from build123d import *

# Parameters (mm, degrees)
EXTRUDE_3_DEPTH    = 3
SKETCH1_W          = 15
SKETCH1_H          = 40
SKETCH1_W_2        = 3
SKETCH1_H_2        = 20
CUT_EXTRUDE1_DEPTH = 10
FILLET1_R          = 15


with BuildPart() as part:
    # Эскиз4 → Бобышка-Вытянуть3 (new body)
    with BuildSketch(Plane(origin=(0, 0, 0), x_dir=(1, 0, 0), z_dir=(0, 1, 0))):
        Polygon((98, 0), (98, 110), (58, 110), (58, 107), (55, 107), (52, 107), (52, 110), (0, 110), (0, 58), (3, 58), (3, 55), (3, 52), (0, 52), (0, 0), (52, 0), (52, 3), (55, 3), (58, 3), (58, 0), align=None)
    extrude(amount=EXTRUDE_3_DEPTH)

    # Sketch1 → Cut-Extrude1 (cut)
    with BuildSketch(Plane(origin=(0, 3, 0), x_dir=(1, 0, 0), z_dir=(0, 1, 0))):
        with Locations((26.5, 55)):
            Rectangle(SKETCH1_W, SKETCH1_H)
        with Locations((55, 55)):
            Rectangle(SKETCH1_W_2, SKETCH1_H_2)
    extrude(amount=-CUT_EXTRUDE1_DEPTH, mode=Mode.SUBTRACT)

    # Fillet1
    fillet1_edges = [part.edges().sort_by_distance(p)[0] for p in [
        (0, 1.5, 0),
        (0, 1.5, -110),
    ]]
    fillet(fillet1_edges, radius=FILLET1_R)


solid = part.part
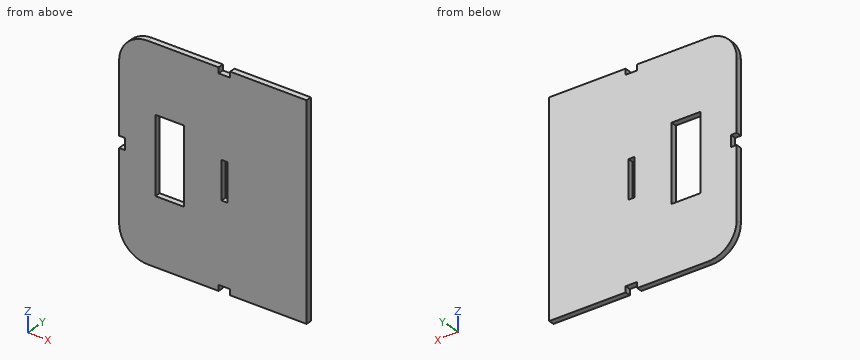
CAD build for the part. Positions are in the model's coordinates, mm. Coordinates: 2 decimals unless noted, no trailing zeros. Write each loop counter-clockwise with the first axis right and the second up, starting at its lowest first coordinate (ties: lowest second). Pieces come first, ordered by that corner, then holes. Notation, with made-up numbers: M 72.5,40 L 98.5,40 A34 cw 98.5,73 Z; hole C 86.5,30 d7. An arc over 180 degrees is marked long. Return JSON: item names as keys, results as strings.
Item 1: Drop flat-ended pins along their axis: pin 1 Ø1.5 at (y, z) = (1.5, -1.5) entering from -X; pin 2 Ø0.9 at (x, y) = (1, 2) entering from -Z; pin 3 Ø1.5 at (x, y) = (54, 2) entering from -Z. Give the stop position or say it passes through.
Findings below:
{"pin 1": "stops at x = 7.1", "pin 2": "stops at z = -101.43", "pin 3": "stops at z = -107"}
Item 2: Slice it at B-B, the plane z = -68. Write the cut outline in (x, y), and give its area (3 significant figures).
Findings below:
{"outline": "M 0,0 L 19,0 L 19,3 L 0,3 Z; M 34,0 L 98,0 L 98,3 L 34,3 Z", "area": "249 mm2"}
Item 3: Slice it at C-C, the plane y = 1.8. Write the cut outline in (x, z), and give its area (3 significant figures).
Findings below:
{"outline": "M 0,-95 A15 ccw 15,-110 L 52,-110 L 52,-107 L 58,-107 L 58,-110 L 98,-110 L 98,0 L 58,0 L 58,-3 L 52,-3 L 52,0 L 15,0 A15 ccw 0,-15 L 0,-52 L 3,-52 L 3,-58 L 0,-58 Z; hole M 19,-75 L 34,-75 L 34,-35 L 19,-35 Z; hole M 53.5,-65 L 56.5,-65 L 56.5,-45 L 53.5,-45 Z", "area": "9,970 mm2"}
Item 4: Slice it at A-A, the plane z = -50. Write the cut outline in (x, y), and give its area (3 significant figures).
Findings below:
{"outline": "M 0,0 L 19,0 L 19,3 L 0,3 Z; M 34,0 L 53.5,0 L 53.5,3 L 34,3 Z; M 56.5,0 L 98,0 L 98,3 L 56.5,3 Z", "area": "240 mm2"}
Item 5: Probe line 1 (X direction, y = 2.6, z = -54); line 2 (X direction, y = 1.5, z = -50.5); line 3 (Z direction, x = 22, y = 0.5). List the from-to ranges inside material, lowest first. Write a range as from..to.
Findings below:
{"line 1": "x = 3..19, 34..53.5, 56.5..98", "line 2": "x = 0..19, 34..53.5, 56.5..98", "line 3": "z = -110..-75, -35..0"}
